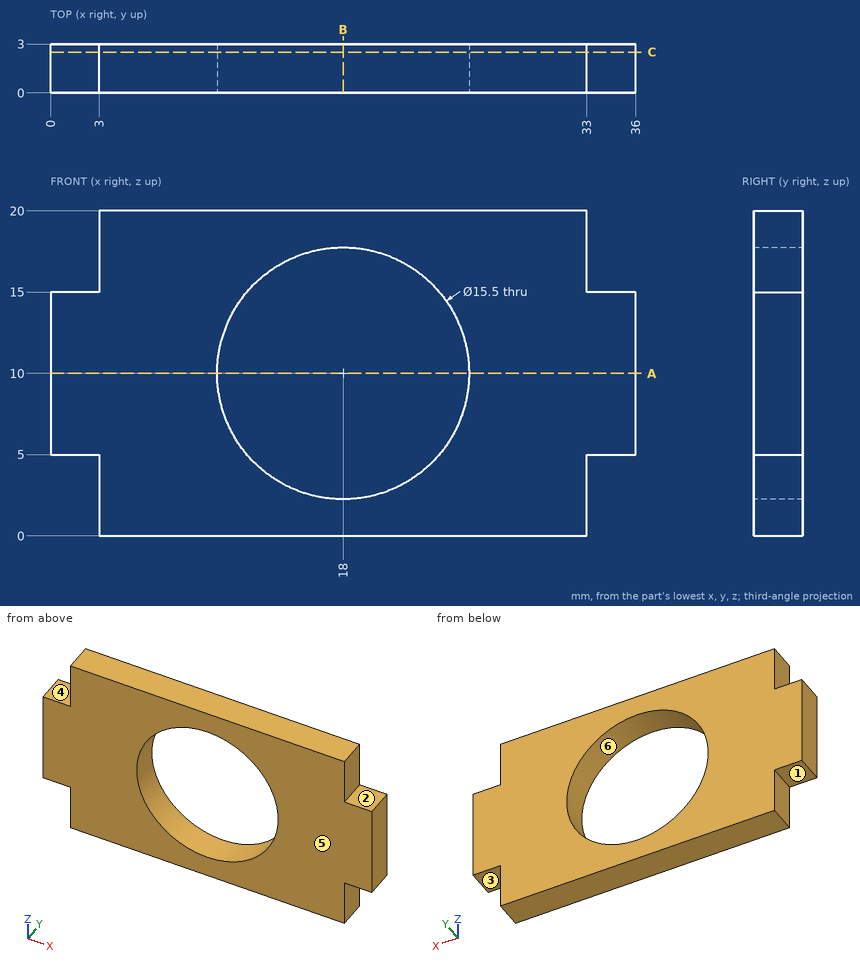
Part print with two shaded views. Sizes in mm from the minimum x, y, z corner. A direction names the side the tool comes from. Round coordinates to 2 decimals unless told otherwise and drop trailing zeros. Order: outer loops, then holes, each group sorted by start corner. A loop starts at its lowest first (then second) coordinate and runs counter-clockwise, first axis right, second up. Notation, with made-up numbers: (53, -25) - (101, -25) arc R27 ccw to (101, 11) - close; hole circle Ø1 at (49, 30.25). An arc over 180 degrees is marked (long way). Return JSON: item names as keys, results as strings.
(1) Cut at A-A (z = 10). Give the cut face in (x, y), then the cut area to 3 significant figures.
Answer key:
{"outline": "(0, 0) - (10.25, 0) - (10.25, 3) - (0, 3) - close; (25.75, 0) - (36, 0) - (36, 3) - (25.75, 3) - close", "area": "61.5 mm^2"}
(2) Pull direction X, two halves, no side cores. Call the marked faces 5 and 6: +X half, -X half, draft (parallel to the pull), parting line (faces both ways), or undercut.
Answer key:
{"face 5": "draft", "face 6": "undercut"}
(3) Cut at B-B (x = 18). Give the cut face in (y, z).
Answer key:
{"outline": "(0, 0) - (3, 0) - (3, 2.25) - (0, 2.25) - close; (0, 17.75) - (3, 17.75) - (3, 20) - (0, 20) - close"}
(4) Wall check: probe 1 along X at (y, z) = (1.7, 10); probe 2 along X at (y, z) = (1, 18.75); probe 3 along Z at (x, y) = (2.5, 0.95). Give the ranges that are in metal, low to high. Write a range as from..to.
Answer key:
{"probe 1": "x = 0..10.25, 25.75..36", "probe 2": "x = 3..33", "probe 3": "z = 5..15"}
(5) Cut at C-C (y = 2.5). Give the cut face in (x, z), then the cut area to 3 significant figures.
Answer key:
{"outline": "(0, 5) - (3, 5) - (3, 0) - (33, 0) - (33, 5) - (36, 5) - (36, 15) - (33, 15) - (33, 20) - (3, 20) - (3, 15) - (0, 15) - close; hole circle Ø15.5 at (18, 10)", "area": "471 mm^2"}
(6) Tool access for the marked faces 1, 2, 3 and 4: list every direction of +Z, -Z, +X, -X, +Y, -Y with a clear straight run to the whole face (end or side of a thin tool).
Answer key:
{"face 1": "-Z, -X, +Y, -Y", "face 2": "+Z, +X, +Y, -Y", "face 3": "-Z, +X, +Y, -Y", "face 4": "+Z, -X, +Y, -Y"}
(7) Pin check, flat tips, straight feed: pin 1 Ø1 at (y, z) = (1, 3.5) entering from -X; pin 2 Ø1.5 at (x, y) = (35, 1.5) entering from -Z; pin 3 Ø1.5 at (y, z) = (1.5, 3) entering from +X. Stop position of each tip, or through.
Answer key:
{"pin 1": "stops at x = 3", "pin 2": "stops at z = 5", "pin 3": "stops at x = 33"}
